```python
from build123d import *

# Parameters (mm, degrees)
SKETCH1_W           = 5
SKETCH1_H           = 30
SKETCH1_R           = 1.55
BOSS_EXTRUDE1_DEPTH = 3
FILLET1_R           = 2.5


with BuildPart() as part:
    # Sketch1 → Boss-Extrude1 (new body)
    with BuildSketch(Plane(origin=(0, 0, 0), x_dir=(1, 0, 0), z_dir=(0, 1, 0))):
        Rectangle(SKETCH1_W, SKETCH1_H)
        with Locations(Location((0, 12, 0), (0, 0, 270))):
            Circle(SKETCH1_R, mode=Mode.SUBTRACT)
        with Locations(Location((0, -12, 0), (0, 0, 270))):
            Circle(SKETCH1_R, mode=Mode.SUBTRACT)
    extrude(amount=BOSS_EXTRUDE1_DEPTH)

    # Fillet1
    fillet1_edges = [part.edges().sort_by_distance(p)[0] for p in [
        (-2.5, 1.5, 15),
        (-2.5, 1.5, -15),
    ]]
    fillet(fillet1_edges, radius=FILLET1_R)


solid = part.part
```
Source: CAD feature listing. Evaluate the final solid. Frame: model axes, mm. Coordinates: 2 decimals unless noted, no trailing zeros. Loops run counter-clockwise (first coordinate to the right, second up) from the corner with the lowest first, then second, coordinate; pieces in that order, holes last. Notation, with made-up numbers: (-11, 75) - (44, 75) arc R18 cw to (44, 102) - close; hole circle Ø9 at (71.5, 58.5). An arc over 180 degrees is marked (long way). Answer as CSV lines item,"result".
1. Mould query, pull axis Z, two halves, no side actions, for faces 1 (the flat face through (1, 1, -15)), 2 (the flat face through (0, 0, 0)), 3 (the cylindrical face through (0.07, 1.48, -13.55)). Classes: released by +Z, released by -Z, zero draft, split by the parting line, or undercut.
Established:
face 1,"released by -Z"
face 2,"zero draft"
face 3,"undercut"
2. Ray query, line 1 (X direction, y = 1.3, z = -12); line 2 (Z direction, x = 0.15, y = 0.55); line 3 (Z direction, x = 0.95, y = 1.05). Return the intervals inside material, ascending.
Established:
line 1,"x = -2.5 to -1.55, 1.55 to 2.5"
line 2,"z = -15 to -13.54, -10.46 to 10.46, 13.54 to 15"
line 3,"z = -15 to -13.22, -10.78 to 10.78, 13.22 to 15"
3. Section C-C (x = -1.25). Return loops of the section in (y, z).
Established:
outline,"(0, -14.67) - (3, -14.67) - (3, -12.92) - (0, -12.92) - close; (0, -11.08) - (3, -11.08) - (3, 11.08) - (0, 11.08) - close; (0, 12.92) - (3, 12.92) - (3, 14.67) - (0, 14.67) - close"
4. Section A-A (z = -12). Return loops of the section in (x, y), then the cut area to 3 significant figures.
Established:
outline,"(-2.5, 0) - (-1.55, 0) - (-1.55, 3) - (-2.5, 3) - close; (1.55, 0) - (2.5, 0) - (2.5, 3) - (1.55, 3) - close"
area,"5.70 mm2"
5. Section B-B (y = 2.05). Return loops of the section in (x, z).
Established:
outline,"(-2.5, -12.5) arc R2.5 ccw to (0, -15) - (2.5, -15) - (2.5, 15) - (0, 15) arc R2.5 ccw to (-2.5, 12.5) - close; hole circle Ø3.1 at (0, -12); hole circle Ø3.1 at (0, 12)"
